Autodesk Inventor part; units mm, degrees
ref_plane "YZ Plane" through (0, 0, 0) normal (1, 0, 0) x (0, 1, 0)
ref_plane "XZ Plane" through (0, 0, 0) normal (0, 1, 0) x (-1, 0, 0)
ref_plane "XY Plane" through (0, 0, 0) normal (0, 0, 1) x (1, 0, 0)
sketch "Sketch1" plane through (0, 0, 0) normal (0, 0, 1) x (1, 0, 0)
  line L0 (0.6985, 3.9665) -> (0.6985, 6.5405)
  line L1 (0.3175, 6.1595) -> (0.3175, 3.9665)
  line L2 (-1.651, 6.35) -> (-1.651, 6.731)
  line L3 (-1.27, 6.731) -> (-1.27, 9.906)
  line L4 (-1.27, 9.906) -> (-1.651, 9.906)
  line L5 (-1.651, 9.906) -> (-1.651, 6.35)
  line L6 (-0.0635, 2.0785) -> (-0.0635, 0.1905)
  line L7 (-0.0635, 0.1905) -> (0.3175, 0.1905)
  line L8 (0.3175, 0.1905) -> (0.3175, 2.0785)
  line L9 (0.6985, 3.9665) -> (0.3175, 2.0785)
  line L10 (0.3175, 3.9665) -> (-0.0635, 2.0785)
  line L11 (-1.27, 6.731) -> (0.6985, 6.5405)
  line L12 (-1.651, 6.35) -> (0.3175, 6.1595)
  point P0 (0, 0)
  dimension "d3" = 0.381
  dimension "d4" = 0.381
extrude "Extrusion1" add sketch "Sketch1" along normal blind 1.651
fillet "Fillet1" radius 0.127 2 edges at (0.3175, 6.1595, 0.8255) (-1.27, 6.731, 0.8255)
fillet "Fillet2" radius 0.508 2 edges at (-1.651, 6.35, 0.8255) (0.6985, 6.5405, 0.8255)
fillet_without_effect "Fillet3"
sketch "Sketch3" plane through (-0.0635, 0.1905, 0) normal (-1, 0, 0) x (0, 0, 1)
  line L0 (0, 0) -> (0.7874, 0)
  line L1 (0.7874, 0) -> (0.7874, 2.54)
  line L2 (0.7874, 2.54) -> (0, 2.54)
  line L3 (0, 2.54) -> (0, 0)
  point P0 (0, -0.1905)
  dimension "d18" = 0.7874
  dimension "d19" = 2.54
extrude "Extrusion3" cut sketch "Sketch3" against normal through all
sketch "Sketch4" plane through (0, 0, 1.651) normal (0, 0, 1) x (1, 0, 0)
  line L0 (-1.651, 9.906) -> (-0.889, 9.906)
  line L1 (-0.889, 9.906) -> (-0.889, 9.525)
  line L2 (-0.889, 9.525) -> (-1.651, 9.525)
  line L3 (-1.651, 9.525) -> (-1.651, 9.906)
  point P0 (0, 0)
  dimension "d22" = 0.762
  dimension "d23" = 0.381
extrude "Extrusion4" add sketch "Sketch4" against normal blind 1.651
fillet "Fillet4" radius 0.381 1 edges at (-1.651, 9.906, 0.8255)
fillet "Fillet5" radius 0.508 2 edges at (0.127, 0.1905, 1.651) (0.127, 0.1905, 0.7874)
properties part number "pin_1"
Model file for the job. Use its own axes, mm. A direction names the side the tool comes from. Give positions to 0.01 mm unless a question says otherwise; leave off trailing zeros. Order: outer loops, then holes, each group sorted by start corner. A loop starts at its lowest first (then second) coordinate and runs counter-clockwise, first axis right, second up. Notation, with made-up numbers: (76, -27) - (108, -27) arc R28 ccw to (108, 4) - close; hole circle Ø1 at (74, 61). An arc over 180 degrees is marked (long way). Write item = value, one per line. Start each with the question number.
1. Cut at B-B, the plane x = -0.2. List the corners of the cut face in (y, z), and give its area (3 significant figures).
2. Drop flat-ended pins along their axis: P1, Ø0.7, axis at y = 1, z = 1.5, coming from the +X side; P2, Ø0.8, axis at y = 5, z = 1, coming from the -X side. Give the stop position or say it passes through.
3. Cut at A-A, the plane y = 1.75. List the corners of the cut face in (x, z), and give its area (3 significant figures).
4. Which spindle directions (+Z, -Z, +X, -X, +Y, -Y) get a long thin tool onto all of the face, cutting with end or side? Do faces 1 (the flat face through (-0.468, 6.653, 0.814)), 2 (the flat face through (-1.651, 8, 1)), 3 (the flat face through (0.318, 1, 1)), 4 (the flat face through (-0.064, 1, 1)), 5 (the flat face through (-0.5, 6.24, 0.81)). Say none if no direction does.
5. Probe line 1 along X through (y, z) = (7, 1.5); line 2 along Y through (x, z) = (-0.95, 0.25) (3 decimals); line 3 along X through (y, z) = (5.25, 0.15). List the from-to ranges inside material, lowest first.
6. Two-plate mould, pull along Y, no slides. Class faces 6 (the flat face through (0.698, 5, 1)), 7 (the flat face through (0.318, 5, 1)), 8 (the flat face through (0.553, 3.245, 0.814)): pulls with the +Y half, pulls with the -Y half, needs draft (parallel to the pull), parting line crosses it, or undercut.
Taken from the geometry:
q1.outline = (6.21, 0) - (6.63, 0) - (6.63, 1.65) - (6.21, 1.65) - close
q1.area = 0.690 mm²
q2.P1 = 0.32
q2.P2 = 0.32
q3.outline = (-0.06, 0.79) - (0.32, 0.79) - (0.32, 1.65) - (-0.06, 1.65) - close
q3.area = 0.329 mm²
q4.face_1 = +Z, -Z, +X
q4.face_2 = +Z, -Z, -X, +Y, -Y
q4.face_3 = +Z, -Z, +X, -Y
q4.face_4 = +Z, -Z, -X, -Y
q4.face_5 = +Z, -Z, -X
q5.line_1 = -1.65 to -1.27
q5.line_2 = 6.282 to 6.7, 9.525 to 9.906
q5.line_3 = 0.32 to 0.7
q6.face_6 = needs draft
q6.face_7 = undercut
q6.face_8 = pulls with the -Y half
